```python
from build123d import *

# Parameters (mm, degrees)
SKETCH_1_W      = 6
SKETCH_1_H      = 6
EXTRUDE_1_DEPTH = 0.2
SKETCH_2_W      = 4
SKETCH_2_H      = 4
EXTRUDE_2_DEPTH = 0.2
SKETCH_3_W      = 0.5
SKETCH_3_H      = 4.4
SKETCH_3_W_2    = 4.4
SKETCH_3_H_2    = 0.5
EXTRUDE_3_DEPTH = 0.3
CHAMFER_1_SIZE  = 0.05
CHAMFER_2_SIZE  = 0.1


with BuildPart() as part:
    # 草图1 → 凸台-拉伸1 (new body)
    with BuildSketch(Plane(origin=(0, 0, 0), x_dir=(1, 0, 0), z_dir=(0, 1, 0))):
        Rectangle(SKETCH_1_W, SKETCH_1_H)
    extrude(amount=EXTRUDE_1_DEPTH)

    # 草图2 → 凸台-拉伸2 (add)
    with BuildSketch(Plane(origin=(0, 0.2, 0), x_dir=(1, 0, 0), z_dir=(0, 1, 0))):
        Rectangle(SKETCH_2_W, SKETCH_2_H)
    extrude(amount=EXTRUDE_2_DEPTH)

    # 草图3 → 凸台-拉伸3 (add)
    with BuildSketch(Plane(origin=(0, 0.2, 0), x_dir=(1, 0, 0), z_dir=(0, 1, 0))):
        with Locations((-2.75, 0)):
            Rectangle(SKETCH_3_W, SKETCH_3_H)
        with Locations((0, -2.75)):
            Rectangle(SKETCH_3_W_2, SKETCH_3_H_2)
        with Locations((2.75, 0)):
            Rectangle(SKETCH_3_W, SKETCH_3_H)
        with Locations((0, 2.75)):
            Rectangle(SKETCH_3_W_2, SKETCH_3_H_2)
    extrude(amount=EXTRUDE_3_DEPTH)

    # 倒角1
    chamfer_1_edges = [part.edges().sort_by_distance(p)[0] for p in [
        (0, 0, 3),
        (-3, 0, 0),
        (0, 0, -3),
        (3, 0, 0),
    ]]
    chamfer(chamfer_1_edges, length=CHAMFER_1_SIZE)

    # 倒角2
    chamfer_2_edges = [part.edges().sort_by_distance(p)[0] for p in [
        (3, 0.125, 3),
        (3, 0.125, -3),
        (-3, 0.125, -3),
        (-3, 0.125, 3),
    ]]
    chamfer(chamfer_2_edges, length=CHAMFER_2_SIZE - 0.0001)  # a hair under: the kernel refuses the full size


solid = part.part
```
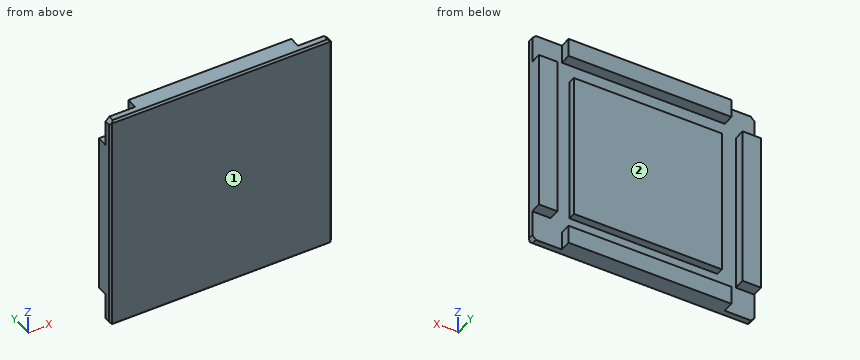
Here's how the part is built. I have some questions about the finished solid (model axes, mm). Face numbers are marked on the shaded views. Give positions to 0.01 mm unless a question says otherwise; leave off trailing zeros. Write each loop counter-clockwise with the first axis right and the second up, starting at its lowest first coordinate (ties: lowest second). Pieces come first, ordered by that corner, then holes.
(1) Imagine slicing it at B-B, the plane x = 1. Write out the boundary of the cut face in (y, z), and give its area (3 significant figures).
Output values:
outline: (0, -2.95) - (0.05, -3) - (0.5, -3) - (0.5, -2.5) - (0.2, -2.5) - (0.2, -2) - (0.4, -2) - (0.4, 2) - (0.2, 2) - (0.2, 2.5) - (0.5, 2.5) - (0.5, 3) - (0.05, 3) - (0, 2.95) - close
area: 2.30 mm2
(2) Imagine slicing it at A-A, the plane z = -1.15. Write out the boundary of the cut face in (x, y).
Output values:
outline: (-3, 0.05) - (-2.95, 0) - (2.95, 0) - (3, 0.05) - (3, 0.5) - (2.5, 0.5) - (2.5, 0.2) - (2, 0.2) - (2, 0.4) - (-2, 0.4) - (-2, 0.2) - (-2.5, 0.2) - (-2.5, 0.5) - (-3, 0.5) - close
(3) If I drill on L1, parallel to Z at x = -1.85, y = 0.35; L2, parallel to X at y = 0.45, z = 2.05, over which ranges is the centre line in solid material (lowest first)?
Output values:
L1: z = -3 to -2.5, -2 to 2, 2.5 to 3
L2: x = -3 to -2.5, 2.5 to 3
(4) Will this pin go through, and if not, where does the flat tip stop? pin 1 (3 mm diameter, centred on x = 0, z = 0.5, fed in from +Y).
Output values:
pin 1: stops at y = 0.4
(5) Imagine slicing it at C-C, the plane z = -2.1. Write out the boundary of the cut face in (x, y).
Output values:
outline: (-3, 0.05) - (-2.95, 0) - (2.95, 0) - (3, 0.05) - (3, 0.5) - (2.5, 0.5) - (2.5, 0.2) - (-2.5, 0.2) - (-2.5, 0.5) - (-3, 0.5) - close
(6) Thinking about a two-plate mould opening in X: for the marked faces 1 and 2, which applies, pulls with the +X half, pulls with the -X half, needs draft (parallel to the pull), parting line crosses it, or undercut?
Output values:
face 1: needs draft
face 2: undercut
